Verification items for the finished model (mm, model axes). A direction names the side the tool comes from. Round coordinates to 2 decimals unless told otherwise and drop trailing zeros. Write each loop counter-clockwise with the first axis right and the second up, starting at its lowest first coordinate (ties: lowest second). Pieces come first, ordered by that corner, then holes. Notation, with made-up numbers: M 24,17 L 55,17 A8 ccw 55,24 Z; hole C 66,33.5 d10. An arc over 180 degrees is marked long. One line per item, written item: value. Start each with the question number.
Item 1: Draft check along Y on faces 4 (the face through (49, -6, 8.7)), 5 (the face through (49, 0, -4)), 6 (the face through (49, -10, 7)), 7 (the face through (49, 10, -7)). Enter one of: +Y half, -Y half, draft (parallel to the pull), parting line (faces both ways), or undercut.
Item 2: Section check C-C, the plane z = 5.5. Record the cut outline in (x, y), then the cut area to 3 significant figures.
Item 3: Section check D-D, the plane y = 6. Record the cut outline in (x, z).
Item 4: Thickness scan on probe 1 along Z at (x, y) = (19, -9); probe 2 along Z at (x, y) = (85.5, 0); probe 3 along Y at (x, z) = (43, 6.5). Record the ranges inside material, lowest first. Write a range as from..to.
Item 5: Section check A-A, the plane y = 0. Record the cut outline in (x, z), then the cut area to 3 significant figures.
Item 6: Tool access check on faces 1 (the face through (49, -4, 0)), 2 (the face through (49.3, -6.29, -5.37)), 3 (the face through (49, 7, -10)). Record the directions out of +Z, -Z, +X, -X, +Y, -Y that give a thin tool (end or side, any length) a straight path to the whole face; none if there is none.
Item 7: Gauge pin test, flat ends, axial feed: pin 1 (2 mm diameter, centred on x = 79, y = -1.5, fed in from +Z); pin 2 (5 mm diameter, centred on x = 76, z = 1, fed in from -Y); pin 3 (1.5 mm diameter, centred on x = 54, z = -1, fed in from -Y). Record the tip position at first contact, or that the pin passes through.
from build123d import *

# Parameters (mm, degrees)
SKETCH1_R                                   = 3
QUADRADO_PF20_01_PERFIL_2020_B_SICO_1_DEPTH = 100


with BuildPart() as part:
    # Sketch1 → Quadrado PF20-01 - PERFIL 2020 BÁSICO(1) (new body)
    with BuildSketch(Plane.YZ):
        with BuildLine():
            Line((8.187867966, -7.26862915), (4.439339828, -3.520101013))
            ThreePointArc((4.439339828, -3.520101013), (4.114180701, -3.033465989), (4, -2.459440841))
            Line((4, -2.459440841), (4, 2.459440841))
            ThreePointArc((4, 2.459440841), (4.114180701, 3.033465989), (4.439339828, 3.520101013))
            Line((4.439339828, 3.520101013), (8.187867966, 7.26862915))
            ThreePointArc((8.187867966, 7.26862915), (8.51480503, 7.333660975), (8.7, 7.056497116))
            Line((8.7, 7.056497116), (8.7, 4))
            Line((8.7, 4), (10, 4))
            Line((10, 4), (10, 9.5))
            ThreePointArc((10, 9.5), (9.853553391, 9.853553391), (9.5, 10))
            Line((9.5, 10), (4, 10))
            Line((4, 10), (4, 8.7))
            Line((4, 8.7), (7.056497116, 8.7))
            ThreePointArc((7.056497116, 8.7), (7.333660975, 8.51480503), (7.26862915, 8.187867966))
            Line((7.26862915, 8.187867966), (3.520101013, 4.439339828))
            ThreePointArc((3.520101013, 4.439339828), (3.033465989, 4.114180701), (2.459440841, 4))
            Line((2.459440841, 4), (-2.459440841, 4))
            ThreePointArc((-2.459440841, 4), (-3.033465989, 4.114180701), (-3.520101013, 4.439339828))
            Line((-3.520101013, 4.439339828), (-7.26862915, 8.187867966))
            ThreePointArc((-7.26862915, 8.187867966), (-7.333660975, 8.51480503), (-7.056497116, 8.7))
            Line((-7.056497116, 8.7), (-4, 8.7))
            Line((-4, 8.7), (-4, 10))
            Line((-4, 10), (-9.5, 10))
            ThreePointArc((-9.5, 10), (-9.853553391, 9.853553391), (-10, 9.5))
            Line((-10, 9.5), (-10, 4))
            Line((-10, 4), (-8.7, 4))
            Line((-8.7, 4), (-8.7, 7.056497116))
            ThreePointArc((-8.7, 7.056497116), (-8.51480503, 7.333660975), (-8.187867966, 7.26862915))
            Line((-8.187867966, 7.26862915), (-4.439339828, 3.520101013))
            ThreePointArc((-4.439339828, 3.520101013), (-4.114180701, 3.033465989), (-4, 2.459440841))
            Line((-4, 2.459440841), (-4, -2.459440841))
            ThreePointArc((-4, -2.459440841), (-4.114180701, -3.033465989), (-4.439339828, -3.520101013))
            Line((-4.439339828, -3.520101013), (-8.187867966, -7.26862915))
            ThreePointArc((-8.187867966, -7.26862915), (-8.51480503, -7.333660975), (-8.7, -7.056497116))
            Line((-8.7, -7.056497116), (-8.7, -4))
            Line((-8.7, -4), (-10, -4))
            Line((-10, -4), (-10, -9.5))
            ThreePointArc((-10, -9.5), (-9.853553391, -9.853553391), (-9.5, -10))
            Line((-9.5, -10), (-4, -10))
            Line((-4, -10), (-4, -8.7))
            Line((-4, -8.7), (-7.056497116, -8.7))
            ThreePointArc((-7.056497116, -8.7), (-7.333660975, -8.51480503), (-7.26862915, -8.187867966))
            Line((-7.26862915, -8.187867966), (-3.520101013, -4.439339828))
            ThreePointArc((-3.520101013, -4.439339828), (-3.033465989, -4.114180701), (-2.459440841, -4))
            Line((-2.459440841, -4), (2.459440841, -4))
            ThreePointArc((2.459440841, -4), (3.033465989, -4.114180701), (3.520101013, -4.439339828))
            Line((3.520101013, -4.439339828), (7.26862915, -8.187867966))
            ThreePointArc((7.26862915, -8.187867966), (7.333660975, -8.51480503), (7.056497116, -8.7))
            Line((7.056497116, -8.7), (4, -8.7))
            Line((4, -8.7), (4, -10))
            Line((4, -10), (9.5, -10))
            ThreePointArc((9.5, -10), (9.853553391, -9.853553391), (10, -9.5))
            Line((10, -9.5), (10, -4))
            Line((10, -4), (8.7, -4))
            Line((8.7, -4), (8.7, -7.056497116))
            ThreePointArc((8.7, -7.056497116), (8.51480503, -7.333660975), (8.187867966, -7.26862915))
        make_face()
        Circle(SKETCH1_R, mode=Mode.SUBTRACT)
    extrude(amount=QUADRADO_PF20_01_PERFIL_2020_B_SICO_1_DEPTH)


solid = part.part
Response values:
1. face 4: undercut
1. face 5: undercut
1. face 6: -Y half
1. face 7: +Y half
2. outline: M 0,-10 L 100,-10 L 100,-8.7 L 0,-8.7 Z; M 0,-6.42 L 100,-6.42 L 100,-4.58 L 0,-4.58 Z; M 0,4.58 L 100,4.58 L 100,6.42 L 0,6.42 Z; M 0,8.7 L 100,8.7 L 100,10 L 0,10 Z
2. area: 628 mm2
3. outline: M 0,-10 L 100,-10 L 100,-8.7 L 0,-8.7 Z; M 0,-6.92 L 100,-6.92 L 100,-5.08 L 0,-5.08 Z; M 0,5.08 L 100,5.08 L 100,6.92 L 0,6.92 Z; M 0,8.7 L 100,8.7 L 100,10 L 0,10 Z
4. probe 1: z = -10..-4, 4..10
4. probe 2: z = -4..-3, 3..4
4. probe 3: y = -10..-8.7, -7.42..-5.58, 5.58..7.42, 8.7..10
5. outline: M 0,-4 L 100,-4 L 100,-3 L 0,-3 Z; M 0,3 L 100,3 L 100,4 L 0,4 Z
5. area: 200 mm2
6. face 1: +X, -X, -Y
6. face 2: +X, -X
6. face 3: -Z, +X, -X, +Y, -Y
7. pin 1: stops at z = 4
7. pin 2: stops at y = -4.42
7. pin 3: stops at y = -4
